```python
from build123d import *

# Parameters (mm, degrees)
ESQUISSE1_W              = 350
ESQUISSE1_H              = 250
BOSS_EXTRU_1_DEPTH       = 5
ENL_V_MAT_EXTRU_1_DEPTH  = 5
CONG_1_R                 = 5
ESQUISSE8_W              = 85
ESQUISSE8_H              = 60
ENL_V_MAT_EXTRU_12_DEPTH = 5
ESQUISSE9_R              = 2.5
ENL_V_MAT_EXTRU_14_DEPTH = 5
ESQUISSE10_W             = 80
ESQUISSE10_H             = 67
ENL_V_MAT_EXTRU_15_DEPTH = 10


with BuildPart() as part:
    # Esquisse1 → Boss.-Extru.1 (new body)
    with BuildSketch(Plane.XY):
        with Locations((0, 125)):
            Rectangle(ESQUISSE1_W, ESQUISSE1_H)
    extrude(amount=BOSS_EXTRU_1_DEPTH)

    # Esquisse2 → Enlèv. mat.-Extru.1 (cut)
    with BuildSketch(Plane.XY):
        Polygon((-61.749658188, 183.853742021), (-75.699374837, 164.324138712), (-116.386048398, 193.386048398), (-126.848335885, 178.738845916), (-151.260340021, 196.175991728), (-116.386048398, 245), (-91.974044262, 227.562854188), (-102.436331748, 212.915651707), align=None)
        Polygon((61.749658188, 183.853742021), (75.699374837, 164.324138712), (116.386048398, 193.386048398), (126.848335885, 178.738845916), (151.260340021, 196.175991728), (116.386048398, 245), (91.974044262, 227.562854188), (102.436331748, 212.915651707), align=None)
        Polygon((61.749658188, 66.146257979), (75.699374837, 85.675861288), (116.386048398, 56.613951602), (126.848335885, 71.261154084), (151.260340021, 53.824008272), (116.386048398, 5), (91.974044262, 22.437145812), (102.436331748, 37.084348293), align=None)
        Polygon((-61.749658188, 66.146257979), (-75.699374837, 85.675861288), (-116.386048398, 56.613951602), (-126.848335885, 71.261154084), (-151.260340021, 53.824008272), (-116.386048398, 5), (-91.974044262, 22.437145812), (-102.436331748, 37.084348293), align=None)
    extrude(amount=ENL_V_MAT_EXTRU_1_DEPTH, mode=Mode.SUBTRACT)

    # Congé1
    cong_1_edges = [part.edges().sort_by_distance(p)[0] for p in [
        (-175, 250, 2.5),
        (175, 250, 2.5),
        (175, 0, 2.5),
        (-175, 0, 2.5),
    ]]
    fillet(cong_1_edges, radius=CONG_1_R)

    # Esquisse8 → Enlèv. mat.-Extru.12 (cut)
    with BuildSketch(Plane.XY):
        with Locations((0, 220)):
            Rectangle(ESQUISSE8_W, ESQUISSE8_H)
        with Locations((0, 30)):
            Rectangle(ESQUISSE8_W, ESQUISSE8_H)
    extrude(amount=ENL_V_MAT_EXTRU_12_DEPTH, mode=Mode.SUBTRACT)

    # Esquisse9 → Enlèv. mat.-Extru.14 (cut)
    with BuildSketch(Plane.XY):
        with Locations((-64.5, 35)):
            Circle(ESQUISSE9_R)
        with Locations(Location((64.5, 35, 0), (0, 0, 180))):
            Circle(ESQUISSE9_R)
        with Locations((64.5, 215)):
            Circle(ESQUISSE9_R)
        with Locations(Location((-64.5, 215, 0), (0, 0, 180))):
            Circle(ESQUISSE9_R)
    extrude(amount=ENL_V_MAT_EXTRU_14_DEPTH, mode=Mode.SUBTRACT)

    # Esquisse10 → Enlèv. mat.-Extru.15 (cut)
    with BuildSketch(Plane.XY):
        with Locations((-135, 123.5)):
            Rectangle(ESQUISSE10_W, ESQUISSE10_H)
    extrude(amount=ENL_V_MAT_EXTRU_15_DEPTH, mode=Mode.SUBTRACT)


solid = part.part
```
CAD build for the part. Positions are in the model's coordinates, mm. Coordinates: 2 decimals unless noted, no trailing zeros. Order: outer loops, then holes, each group sorted by start corner. A loop starts at its lowest first (then second) coordinate and runs counter-clockwise, first axis right, second up. Notation, with made-up numbers: M -2,9 L 4,9 A21 ccw 4,36 Z; hole C 33.25,-36.75 d11. An arc over 180 degrees is marked long. Write each question's results on one line, items separated by ' | '. Start each with the question number.
Q1. Cut at A-A (x = 147). List the corners of the cut face in (y, z), then the cut area to 3 significant figures.
Q2. Cut at D-D (z = 0.9). Count the separate pieces of the cut face and the enclosed holes in it, then the cut area to 3 significant figures.
Q3. Flat gauge pins, fed straight in: P1, Ø6, axis at x = -64.5, y = 215, coming from the +Z side; P2, Ø4.5, axis at x = -64.5, y = 35, coming from the +Z side. Where does each tip first touch, or does it go through?
Q4. Cut at B-B (y = 82). List the corners of the cut face in (x, z).
Q5. Pull direction X, two halves, no side cores. Call faces 1 (the flat face through (-2, 127, 5)), 2 (the flat face through (104.351, 236.403, 2.465)), 3 (the flat face through (68.627, 75.774, 2.465)): +X half, -X half, draft (parallel to the pull), parting line (faces both ways), or undercut.
Q6. Drill centre lines: probe 1 along Y at (x, z) = (138, 2.25); probe 2 along Y at (x, z) = (-64.5, 3.05); probe 3 along X at (y, z) = (45, 2.95). Where is each one in solid material? Low to high. Write a range as from..to.
Q7. Cut at C-C (y = 134.5). List the corners of the cut face in (x, z).
Found:
1) outline: M 0,0 L 47.86,0 L 47.86,5 L 0,5 Z; M 56.87,0 L 193.13,0 L 193.13,5 L 56.87,5 Z; M 202.14,0 L 250,0 L 250,5 L 202.14,5 Z | area: 1,160 mm²
2) separate pieces: 1 | enclosed holes: 8 | area: 59,800 mm²
3) P1: z = 5 | P2: through
4) outline: M -175,0 L -80.85,0 L -80.85,5 L -175,5 Z; M -73.07,0 L 73.07,0 L 73.07,5 L -73.07,5 Z; M 80.85,0 L 175,0 L 175,5 L 80.85,5 Z
5) face 1: draft | face 2: undercut | face 3: undercut
6) probe 1: 0..35.26, 63.3..186.7, 214.74..250 | probe 2: 0..32.5, 37.5..64.18, 70..180, 185.82..212.5, 217.5..250 | probe 3: -175..-144.96, -91.35..-42.5, 42.5..91.35, 144.96..175
7) outline: M -95,0 L 175,0 L 175,5 L -95,5 Z
